For this review, take the finished solid that the model builds, in its own axes (mm). Coordinates: 2 decimals unless noted, no trailing zeros. Write each loop counter-clockwise with the first axis right and the second up, starting at its lowest first coordinate (ties: lowest second). Pieces come first, ordered by that corner, then holes. Notation, with made-up numbers: (18.25, -21) -> (34.25, -21) arc R9 cw to (34.25, -8) -> close; hole circle Ø8 at (33, -27.5). An arc over 180 degrees is marked (long way). Put each result on its own line as item: value. Start each with the question number.
Item 1: To check wall thickness, follow L1, parallel to Y at x = 185.5, z = -1; L2, parallel to X at y = 12, z = -0.65; L3, parallel to X at y = -9.5, z = -0.9. State the ranges of each line that lie inside material, in increasing order.
Item 2: Insertion check: P1, Ø6, axis at x = 133.5, y = 1, coming from the +Z side. The pin has a flat end and moves straight along its axis. Give the tip position at first contact, or say it passes through.
Item 3: Consider section B-B on z = -0.3. Give the boundary of the cut face in (x, y).
Item 4: Consider section A-A on x = 185.5. Give the boundary of the cut face in (y, z).
Item 5: The part is to be moulded in two halves that separate along Y. For faces 1 (the cylindrical face through (196.65, 21.99, -1.01)), 2 (the cylindrical face through (189.66, 11.28, -0.99)), 3 (the flat face through (-3, 0, -2)), 4 (the cylindrical face through (189.66, -14.72, -0.99)), say which applies: +Y half, -Y half, draft (parallel to the pull), parting line (faces both ways), or undercut.
```python
from build123d import *

# Parameters (mm, degrees)
SKETCH1_W            = 399
SKETCH1_H            = 50
BASE_FLANGE1_DEPTH   = 2
FILLET1_R            = 10
M8_CLEARANCE_HOLE1_D = 9


# Sheet-metal steps are written as plain solids
with BuildPart() as part:
    # Sketch1 → Base-Flange1 (new body)
    with BuildSketch(Plane.XY):
        Rectangle(SKETCH1_W, SKETCH1_H)
    extrude(amount=-BASE_FLANGE1_DEPTH)

    # Fillet1
    fillet1_edges = [part.edges().sort_by_distance(p)[0] for p in [
        (199.5, -25, -1),
        (-199.5, -25, -1),
        (-199.5, 25, -1),
        (199.5, 25, -1),
    ]]
    fillet(fillet1_edges, radius=FILLET1_R)

    # M8 Clearance Hole1 (through all)
    with Locations(Plane(origin=(0, 0, -2), x_dir=(-1, 0, 0), z_dir=(0, 0, -1))):
        with Locations((-185.5, 13), (-185.5, -13)):
            m8_clearance_hole1 = Hole(M8_CLEARANCE_HOLE1_D / 2)

    # Mirror1: M8 Clearance Hole1 across plane
    add(m8_clearance_hole1.mirror(Plane(origin=(0, 0, 0), x_dir=(0, 0, 1), z_dir=(1, 0, 0))), mode=Mode.SUBTRACT)


solid = part.part
```
Return value:
1. L1: -25 to -17.5, -8.5 to 8.5, 17.5 to 25
1. L2: -199.5 to -189.89, -181.11 to 181.11, 189.89 to 199.5
1. L3: -199.5 to -188.33, -182.67 to 182.67, 188.33 to 199.5
2. P1: z = 0
3. outline: (-199.5, -15) arc R10 ccw to (-189.5, -25) -> (189.5, -25) arc R10 ccw to (199.5, -15) -> (199.5, 15) arc R10 ccw to (189.5, 25) -> (-189.5, 25) arc R10 ccw to (-199.5, 15) -> close; hole circle Ø9 at (-185.5, -13); hole circle Ø9 at (-185.5, 13); hole circle Ø9 at (185.5, -13); hole circle Ø9 at (185.5, 13)
4. outline: (-25, -2) -> (-17.5, -2) -> (-17.5, 0) -> (-25, 0) -> close; (-8.5, -2) -> (8.5, -2) -> (8.5, 0) -> (-8.5, 0) -> close; (17.5, -2) -> (25, -2) -> (25, 0) -> (17.5, 0) -> close
5. face 1: +Y half
5. face 2: undercut
5. face 3: draft
5. face 4: undercut
